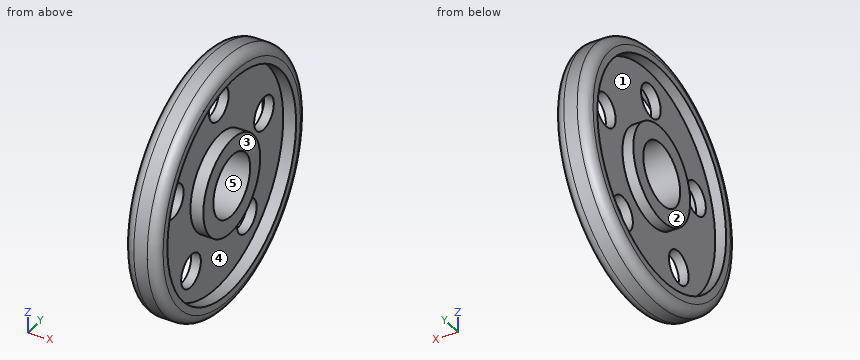
from build123d import *

# Parameters (mm, degrees)
F2_R     = 5.021426
F3_DEPTH = 25
F4_R     = 3


with BuildPart() as f1:
    # F0 (on Front) → F1 (revolve)
    with BuildSketch(Plane.XZ):
        Polygon((0, 14.5267), (0, 9.400629), (10, 9.400629), (10, 14.5267), (6.157054, 14.5267), (6.157054, 32.876216), (10, 32.876216), (10, 38.057327), (0, 38.057327), (0, 32.876216), (3.236998, 32.876216), (3.236998, 14.5267), align=None)
    revolve(axis=Axis((5, 0, 0), (1, 0, 0)))

    # F2 (on face) → F3 (cut)
    with BuildSketch(Plane.YZ.offset(6.157054)):
        with Locations((-23.041325, 7.48658)):
            Circle(F2_R)
        with Locations((0, 24.227083)):
            Circle(F2_R)
        with Locations((23.041325, 7.48658)):
            Circle(F2_R)
        with Locations((14.240322, -19.600122)):
            Circle(F2_R)
        with Locations((-14.240322, -19.600122)):
            Circle(F2_R)
    extrude(amount=-F3_DEPTH, mode=Mode.SUBTRACT)

    # F4
    f4_edges = [f1.edges().sort_by_distance(p)[0] for p in [
        (0, 0, -38.057327),
        (10, 0, -38.057327),
    ]]
    fillet(f4_edges, radius=F4_R)


solid = f1.part
Design review of the part built by this model. Coordinates are the model's own, in mm. Face numbers are marked on the shaded views. A direction names the side the tool comes from. Round coordinates to 2 decimals unless told otherwise and drop trailing zeros. Write each loop counter-clockwise with the first axis right and the second up, starting at its lowest first coordinate (ties: lowest second). Pieces come first, ordered by that corner, then holes. Notation, with made-up numbers: (20.5, 72.25) - (30.5, 72.25) arc R24 ccw to (30.5, 82.25) - close; hole circle Ø3 at (86, 85.25). An arc over 180 degrees is marked (long way). Use a Markdown table: item, result. Add a question column.
1. We need section B-B (y = 0). Count the separate pieces of the cut face and the enclosed holes in it, then the cut area to 3 significant figures.
2. We need section C-C (x = 1). State the section outline as (y, z) points, then the cut area to 3 significant figures.
3. We need section A-A (z = 0). State the section outline as (x, y) points, then the cut area to 3 significant figures.
4. Clearance check with flat-ended pins moving along their axes: pin 1 (4 mm diameter, centred on x = 6, z = -6, fed in from -Y); pin 2 (2 mm diameter, centred on x = 7, z = -7.5, fed in from +Y); pin 3 (24.5 mm diameter, centred on y = 0, z = 0, fed in from -X); pin 4 (5 mm diameter, centred on y = -11.5, z = 15.5, fed in from +X). State where each tip first meets the part, or that it passes through.
5. Mouldability with a two-part tool opening along Y and no side actions: class the marked faces 3, 4 and 5 as +Y half, -Y half, draft (parallel to the pull), parting line (faces both ways), or undercut.
6. For the marked faces 1 and 2, list the 3-axis set-ups (+Z, -Z, +X, -X, +Y, -Y) from which the entire face can be reached by the end or side of a thin tool; tool diameter is ignored.
7. Wall thickness on probe 1 along Z at (x, y) = (7, 0); probe 2 along Z at (x, y) = (2.25, 0); probe 3 along Z at (x, y) = (5.5, 2): over which ranges is each line inside the solid? List them lowest first.
Output:
| question | item | result |
|---|---|---|
| 1 | separate pieces | 3 |
| 1 | enclosed holes | 0 |
| 1 | area | 276 mm2 |
| 2 | outline | circle Ø74.59 at (0, 0); circle Ø29.05 at (0, 0); hole circle Ø65.75 at (0, 0); hole circle Ø18.8 at (0, 0) |
| 2 | area | 1,360 mm2 |
| 3 | outline | (0, -35.06) arc R3 ccw to (3, -38.06) - (7, -38.06) arc R3 ccw to (10, -35.06) - (10, -32.88) - (6.16, -32.88) - (6.16, -14.53) - (10, -14.53) - (10, -9.4) - (0, -9.4) - (0, -14.53) - (3.24, -14.53) - (3.24, -32.88) - (0, -32.88) - close; (0, 9.4) - (10, 9.4) - (10, 14.53) - (6.16, 14.53) - (6.16, 32.88) - (10, 32.88) - (10, 35.06) arc R3 ccw to (7, 38.06) - (3, 38.06) arc R3 ccw to (0, 35.06) - (0, 32.88) - (3.24, 32.88) - (3.24, 14.53) - (0, 14.53) - close |
| 3 | area | 306 mm2 |
| 4 | pin 1 | stops at y = -37.85 |
| 4 | pin 2 | stops at y = 37.5 |
| 4 | pin 3 | stops at x = 0 |
| 4 | pin 4 | stops at x = 6.16 |
| 5 | face 3 | draft |
| 5 | face 4 | undercut |
| 5 | face 5 | undercut |
| 6 | face 1 | -X |
| 6 | face 2 | +Z, -Z, -X, +Y, -Y |
| 7 | probe 1 | z = -38.06 to -32.88, -14.53 to -9.4, 9.4 to 14.53, 32.88 to 38.06 |
| 7 | probe 2 | z = -37.96 to -32.88, -14.53 to -9.4, 9.4 to 14.53, 32.88 to 37.96 |
| 7 | probe 3 | z = -38 to -9.19, 9.19 to 19.62, 28.83 to 38 |
